Part print with two shaded views. Sizes in mm from the minimum x, y, z corner. Give positions to 0.01 mm unless a question says otherwise; leave off trailing zeros. Write each loop counter-clockwise with the first axis right and the second up, starting at its lowest first coordinate (ties: lowest second). Pieces come first, ordered by that corner, then holes. Notation, with made-up numbers: M 5.5,51 L 54.5,51 A29 cw 54.5,76 Z; hole C -31,-9.75 d5. An arc over 180 degrees is marked long. Return JSON: item names as keys, results as strings. Group by question number.
Q1. Wall check: probe 1 along Y at (x, z) = (21, 1.1); probe 2 along Y at (x, z) = (93.5, 1.35) (1 decimal); probe 3 along X at (y, z) = (112, 2.65). Give the ranges that are in metal, low to high.
Q2. Band-saw the part on C-C, the plane y = 194. Give the cut face in (x, z) (1 decimal).
Q3. Band-saw the part on A-A, the plane x = 16. Give the cut face in (y, z) (1 decimal), then the cut area to 3 significant figures.
Q4. Band-saw the part on B-B, the plane z = 2.6. Give the cut face in (x, y), then the cut area to 3 significant figures.
Q5. Flat gauge pins, fed straight in: pin 1 Ø1.5 at (x, z) = (42, 1) entering from -Y; pin 2 Ø1 at (y, z) = (139, 2.5) entering from +X. Where does each tip first touch, or does it go through?
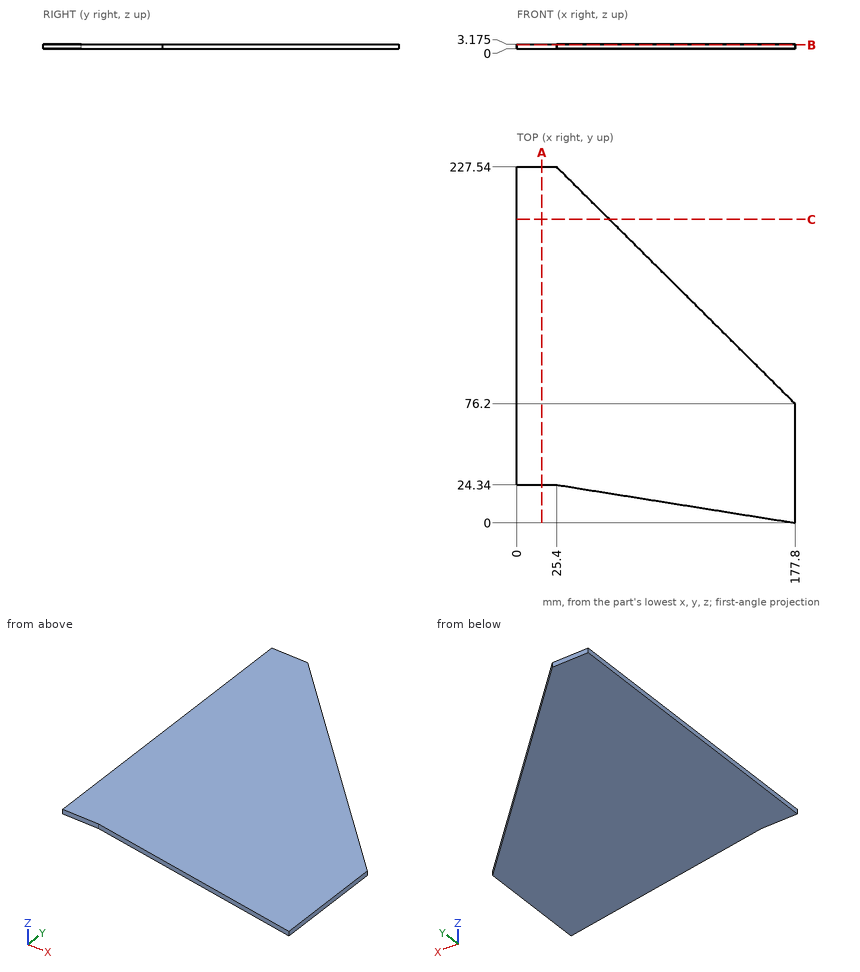
From the geometry:
{
 "1": {"probe 1": "y = 24.34 to 227.54", "probe 2": "y = 13.5 to 159.9", "probe 3": "x = 0 to 141.75"},
 "2": {"outline": "M 0,0 L 59.2,0 L 59.2,3.2 L 0,3.2 Z"},
 "3": {"outline": "M 24.3,0 L 227.5,0 L 227.5,3.2 L 24.3,3.2 Z", "area": "645 mm^2"},
 "4": {"outline": "M 0,24.34 L 25.4,24.34 L 177.8,0 L 177.8,76.2 L 25.4,227.54 L 0,227.54 Z", "area": "26,500 mm^2"},
 "5": {"pin 1": "stops at y = 21.57", "pin 2": "stops at x = 115.06"}
}
